from build123d import *

# Parameters (mm, degrees)
SKETCH2_W           = 52.4
SKETCH2_H           = 51
SKETCH2_R           = 19.896881497
BOSS_EXTRUDE1_DEPTH = 1.6
SKETCH3_W           = 52.4
SKETCH3_H           = 1.8
BOSS_EXTRUDE2_DEPTH = 49.3
SKETCH4_W           = 6
SKETCH4_H           = 6
BOSS_EXTRUDE3_DEPTH = 1
SKETCH5_R           = 1.5
CUT_EXTRUDE1_DEPTH  = 62.006393108
SKETCH6_R           = 1.5
SKETCH6_W           = 43
SKETCH6_H           = 7.2
CUT_EXTRUDE2_DEPTH  = 77.842045782


with BuildPart() as part:
    # Sketch1 → Revolve1 (revolve)
    with BuildSketch(Plane.XY, mode=Mode.PRIVATE) as revolve1_sk:
        with BuildLine():
            Line((4, 15), (5.6, 15))
            ThreePointArc((5.6, 15), (9.845065713, 5.201403427), (19.896881497, 1.596673597))
            Line((19.896881497, 1.596673597), (20, 0))
            ThreePointArc((20, 0), (8.750759907, 4.0341439), (4, 15))
        make_face()
    revolve(revolve1_sk.sketch.rotate(Axis((0, 0, 0), (0, 1, 0)), 90), axis=Axis((0, 0, 0), (0, 1, 0)))

    # Sketch2 → Boss-Extrude1 (add)
    with BuildSketch(Plane(origin=(0, 0, 0), x_dir=(1, 0, 0), z_dir=(0, 1, 0))):
        with Locations((0.5, -0.5)):
            Rectangle(SKETCH2_W, SKETCH2_H)
        with Locations(Location((0, 0, 0), (0, 0, 90))):
            Circle(SKETCH2_R, mode=Mode.SUBTRACT)
    extrude(amount=BOSS_EXTRUDE1_DEPTH)

    # Sketch3 → Boss-Extrude2 (add)
    with BuildSketch(Plane(origin=(0, 1.6, 0), x_dir=(1, 0, 0), z_dir=(0, 1, 0))):
        with Locations((0.5, -25.1)):
            Rectangle(SKETCH3_W, SKETCH3_H)
    extrude(amount=BOSS_EXTRUDE2_DEPTH)

    # Sketch4 → Boss-Extrude3 (add)
    with BuildSketch(Plane(origin=(0, 1.6, 0), x_dir=(1, 0, 0), z_dir=(0, 1, 0))):
        with Locations((22.4, 20.7)):
            Rectangle(SKETCH4_W, SKETCH4_H)
        with Locations((-21.4, 20.7)):
            Rectangle(SKETCH4_W, SKETCH4_H)
    extrude(amount=BOSS_EXTRUDE3_DEPTH)

    # Sketch5 → Cut-Extrude1 (cut, through all)
    with BuildSketch(Plane(origin=(0, 2.6, 0), x_dir=(1, 0, 0), z_dir=(0, 1, 0))):
        with Locations(Location((22.4, 20.7, 0), (0, 0, 270))):
            Circle(SKETCH5_R)
        with Locations(Location((-21.4, 20.7, 0), (0, 0, 270))):
            Circle(SKETCH5_R)
    extrude(amount=-CUT_EXTRUDE1_DEPTH, mode=Mode.SUBTRACT)

    # Sketch6 → Cut-Extrude2 (cut, through all)
    with BuildSketch(Plane.XY.offset(26)):
        with Locations((-20.7, 32.45)):
            Circle(SKETCH6_R)
        with Locations((21.7, 32.45)):
            Circle(SKETCH6_R)
        with Locations((2, 47.3)):
            Rectangle(SKETCH6_W, SKETCH6_H)
    extrude(amount=-CUT_EXTRUDE2_DEPTH, mode=Mode.SUBTRACT)


solid = part.part
For this review, take the finished solid that the model builds, in its own axes (mm). A direction names the side the tool comes from. Coordinates: 2 decimals unless noted, no trailing zeros. Loops run counter-clockwise (first coordinate to the right, second up) from the corner with the lowest first, then second, coordinate; pieces in that order, holes last. Notation, with made-up numbers: (-9, 31.25) - (4, 31.25) arc R10 cw to (4, 41.25) - close; hole circle Ø4 at (0.5, -18.5). An arc over 180 degrees is marked (long way). Use a Markdown table: item, result. Add a question column.
Item 1: For line 1 (X direction, y = 1.65, z = -20.7); line 2 (X direction, y = 0.85, z = -20.7); line 3 (X direction, y = 32, z = 25), list the stretches that pass through material, from the lowest coordinate up.
Item 2: Insertion check: pin 1 Ø2.5 at (x, z) = (22.4, -20.7) entering from +Y; pin 2 Ø1.8 at (x, z) = (-21, -22) entering from +Y; pin 3 Ø0.9 at (x, z) = (12.5, 25) entering from +Y; pin 4 Ø3.5 at (x, z) = (-21.4, -20.7) entering from -Y. Each pin has a flat end and moves straight along its axis. Give the tip position at first contact, or say it passes through.
Item 3: We need section C-C (y = 8.5). Give the boundary of the cut face in (x, z), and give its area (3 significant figures).
Item 4: We need section D-D (x = -21.4). Give the boundary of the cut face in (y, z), and give its area (3 significant figures).
Item 5: Tool access review of faces 1 (the face through (23.5, 47, 25)), 2 (the face through (26.7, 1, 12)), 3 (the face through (4, 15, 2)): name each direction out of +Z, -Z, +X, -X, +Y, -Y from which nothing blocks a thin tool from reaching the whole face with its end or side.
Item 6: We need section A-A (y = 32.45). Give the boundary of the cut face in (x, z), and give its area (3 significant figures).
Item 7: Mouldability with a two-part tool opening along Y and no side actions: class faces 4 (the face through (0, 26, 24.2)), 5 (the face through (-20.895, 33.937, 25.113)), 6 (the face through (12, 0, -17)), 7 (the face through (-23, 2.6, -20)) as pulls with the +Y half, pulls with the -Y half, needs draft (parallel to the pull), parting line crosses it, or undercut.
Results list:
| question | item | result |
|---|---|---|
| 1 | line 1 | x = -24.4 to -22.9, -19.9 to -18.4, 19.4 to 20.9, 23.9 to 25.4 |
| 1 | line 2 | x = -25.7 to -22.9, -19.9 to 20.9, 23.9 to 26.7 |
| 1 | line 3 | x = -25.7 to -22.13, -19.27 to 20.27, 23.13 to 26.7 |
| 2 | pin 1 | passes through |
| 2 | pin 2 | stops at y = 2.6 |
| 2 | pin 3 | stops at y = 43.7 |
| 2 | pin 4 | stops at y = 0 |
| 3 | outline | (-25.7, 24.2) - (26.7, 24.2) - (26.7, 26) - (-25.7, 26) - close; circle Ø14.56 at (0, 0); hole circle Ø10.96 at (0, 0) |
| 3 | area | 166 mm^2 |
| 4 | outline | (0, -25) - (1.6, -25) - (1.6, -23.7) - (2.6, -23.7) - (2.6, -22.2) - (0, -22.2) - close; (0, -19.2) - (2.6, -19.2) - (2.6, -17.7) - (1.6, -17.7) - (1.6, 24.2) - (31.12, 24.2) - (31.12, 26) - (0, 26) - close; (33.78, 24.2) - (50.9, 24.2) - (50.9, 26) - (33.78, 26) - close |
| 4 | area | 164 mm^2 |
| 5 | face 1 | +Z, -Z, +Y |
| 5 | face 2 | +Z, -Z, +X, +Y, -Y |
| 5 | face 3 | -Z, +X, -X, +Y |
| 6 | outline | (-25.7, 24.2) - (-22.2, 24.2) - (-22.2, 26) - (-25.7, 26) - close; (-19.2, 24.2) - (20.2, 24.2) - (20.2, 26) - (-19.2, 26) - close; (23.2, 24.2) - (26.7, 24.2) - (26.7, 26) - (23.2, 26) - close |
| 6 | area | 83.5 mm^2 |
| 7 | face 4 | needs draft |
| 7 | face 5 | undercut |
| 7 | face 6 | pulls with the -Y half |
| 7 | face 7 | pulls with the +Y half |
